Geometry: final body of the model. Coordinates: model frame, mm. A direction names the side the tool comes from. Coordinates: 2 decimals unless noted, no trailing zeros. Loops run counter-clockwise (first coordinate to the right, second up) from the corner with the lowest first, then second, coordinate; pieces in that order, holes last. Notation, with made-up numbers: (71, 13) - (96, 13) arc R15 cw to (96, 34) - close; hole circle Ø4 at (63, -28.75). An arc over 180 degrees is marked (long way). Return JSON: item names as keys, results as strings.
from build123d import *

# Parameters (mm, degrees)
ESQUISSE2_R             = 109
BOSS_EXTRU_1_DEPTH      = 3
ESQUISSE3_W             = 58
ESQUISSE3_H             = 42.41769301
ENL_V_MAT_EXTRU_1_DEPTH = 3


with BuildPart() as part:
    # Esquisse2 → Boss.-Extru.1 (new body)
    with BuildSketch(Plane.XY):
        Circle(ESQUISSE2_R)
    extrude(amount=BOSS_EXTRU_1_DEPTH)

    # Esquisse3 → Enlèv. mat.-Extru.1 (cut)
    with BuildSketch(Plane.XY.offset(3)):
        with Locations((0, -99.780250798)):
            Rectangle(ESQUISSE3_W, ESQUISSE3_H)
        Polygon((-90.279631846, 85.609285361), (-119.279631846, 35.379811942), (-82.544832128, 14.170965437), (-53.544832128, 64.400438856), align=None)
        Polygon((119.279631846, 35.379811942), (90.279631846, 85.609285361), (53.544832128, 64.400438856), (82.544832128, 14.170965437), align=None)
    extrude(amount=-ENL_V_MAT_EXTRU_1_DEPTH, mode=Mode.SUBTRACT)


solid = part.part
Item 1: Section query C-C, the plane z = 1.4. Return loops of the section in (x, y), and give its area (3 significant figures).
Worked out:
{"outline": "(-105.49, 27.42) arc R109 ccw to (-29, -105.07) - (-29, -78.57) - (29, -78.57) - (29, -105.07) arc R109 ccw to (105.49, 27.42) - (82.54, 14.17) - (53.54, 64.4) - (76.49, 77.65) arc R109 ccw to (-76.49, 77.65) - (-53.54, 64.4) - (-82.54, 14.17) - close", "area": "32,300 mm^2"}
Item 2: Section query B-B, the plane y = 21.5. Return loops of the section in (x, z).
Worked out:
{"outline": "(-106.86, 0) - (-95.24, 0) - (-95.24, 3) - (-106.86, 3) - close; (-78.31, 0) - (78.31, 0) - (78.31, 3) - (-78.31, 3) - close; (95.24, 0) - (106.86, 0) - (106.86, 3) - (95.24, 3) - close"}
Item 3: Reachability of faces 4 (the face through (-68.25, 38.93, 1.52)), 5 (the face through (-64.859, 70.933, 1.521)), 6 (the face through (-2, 3, 0)), 7 (the face through (-94.2, 20.9, 1.5)), 8 (the face through (-2, 3, 3)) from +Z, -Z, +X, -X, +Y, -Y: full face, straight path, thin tool, end or side. Return the list, or none.
Worked out:
{"face 4": "+Z, -Z", "face 5": "+Z, -Z, -X", "face 6": "-Z, +X, -X, +Y, -Y", "face 7": "+Z, -Z, +Y", "face 8": "+Z, +X, -X, +Y, -Y"}
Item 4: Mould query, pull axis Y, two halves, no side actions, for faces 1 (the face through (65.18, 71.12, 1.52)), 2 (the face through (-94.985, -53.469, 1.479)), 3 (the face through (93.859, 20.703, 1.521)). Classes: +Y half, -Y half, draft (parallel to the pull), parting line (faces both ways), or undercut.
Worked out:
{"face 1": "undercut", "face 2": "parting line", "face 3": "+Y half"}
Item 5: Ray query, probe 1 along Y at (x, z) = (2, 1.65); probe 2 along Y at (x, z) = (67, 1.45); probe 3 along X at (y, z) = (20.5, 2.8). Return the intervals inside material, ascending. Write a range as from..to.
Worked out:
{"probe 1": "-78.57..108.98", "probe 2": "-85.98..41.1, 72.17..85.98", "probe 3": "-107.05..-93.51, -78.89..78.89, 93.51..107.05"}
Item 6: Section query A-A, the plane x = -71.5. Return loops of the section in (y, z).
Worked out:
{"outline": "(-82.27, 0) - (33.3, 0) - (33.3, 3) - (-82.27, 3) - close; (74.77, 0) - (82.27, 0) - (82.27, 3) - (74.77, 3) - close"}
Item 7: Section query D-D, the plane x = 59.5. Return loops of the section in (y, z), and give its area (3 significant figures).
Worked out:
{"outline": "(-91.33, 0) - (54.09, 0) - (54.09, 3) - (-91.33, 3) - close; (67.84, 0) - (91.33, 0) - (91.33, 3) - (67.84, 3) - close", "area": "507 mm^2"}
Item 8: First-contact query: pin 1 Ø1 at (y, z) = (75.5, 0.5) entering from +X; pin 2 Ø1 at (y, z) = (-67.5, 1) entering from +X; pin 3 Ø0.9 at (y, z) = (-93, 2) entering from +X. Flat tips, straight axial feed; report the tip coordinate or a pass-through.
Worked out:
{"pin 1": "x = 73.64", "pin 2": "x = 85.98", "pin 3": "x = 57.58"}
